Could you check a few things on this model? Use its own coordinates, in mm. A direction names the side the tool comes from. Coordinates: 2 decimals unless noted, no trailing zeros. Order: outer loops, then holes, each group sorted by start corner. A loop starts at its lowest first (then second) coordinate and runs counter-clockwise, first axis right, second up. Notation, with made-up numbers: (-30, 66) - (5, 66) arc R24 ccw to (5, 101) - close; hole circle Ø7 at (79.25, 70). An arc over 180 degrees is marked (long way). One line per item, written item: value. Start each with the question number.
from build123d import *

# Parameters (mm, degrees)
SKETCH1_W             = 15
SKETCH1_H             = 15
BOSS_EXTRUDE1_DEPTH   = 10
SKETCH2_R             = 6
CUT_EXTRUDE1_DEPTH    = 4
SKETCH3_R             = 5
CUT_EXTRUDE2_DEPTH    = 3.5
BOSS_EXTRUDE2_DEPTH   = 6.5
M4_TAPPED_HOLE1_D     = 3.3
M4_TAPPED_HOLE1_DEPTH = 2.5
M2_5_TAPPED_HOLE1_D   = 2.05
SKETCH10_R            = 0.25
CUT_EXTRUDE3_DEPTH    = 0.25
CUT_EXTRUDE4_REACH    = 23.5


with BuildPart() as part:
    # Sketch1 → Boss-Extrude1 (new body)
    with BuildSketch(Plane(origin=(0, 0, 0), x_dir=(1, 0, 0), z_dir=(0, 1, 0))):
        Rectangle(SKETCH1_W, SKETCH1_H)
    extrude(amount=BOSS_EXTRUDE1_DEPTH)

    # Sketch2 → Cut-Extrude1 (cut)
    with BuildSketch(Plane.XZ):
        Circle(SKETCH2_R)
    extrude(amount=-CUT_EXTRUDE1_DEPTH, mode=Mode.SUBTRACT)

    # Sketch3 → Cut-Extrude2 (cut)
    with BuildSketch(Plane.XZ.offset(-4)):
        Circle(SKETCH3_R)
    extrude(amount=-CUT_EXTRUDE2_DEPTH, mode=Mode.SUBTRACT)

    # Sketch4 → Boss-Extrude2 (add)
    with BuildSketch(Plane.XY.offset(7.5)):
        with BuildLine():
            ThreePointArc((5.823428515, 4.483331092), (0, 5.25), (-5.823428515, 4.483331092))
            ThreePointArc((-5.823428515, 4.483331092), (-6.707311991, 2.952400002), (-5.176380902, 2.068516526))
            ThreePointArc((-5.176380902, 2.068516526), (0, 2.75), (5.176380902, 2.068516526))
            ThreePointArc((5.176380902, 2.068516526), (6.707311991, 2.952400002), (5.823428515, 4.483331092))
        make_face()
    boss_extrude2 = extrude(amount=BOSS_EXTRUDE2_DEPTH)

    # Mirror1: Boss-Extrude2 across plane
    add(boss_extrude2.mirror(Plane.XY))

    # M4 Tapped Hole1
    with Locations(Plane(origin=(0, 10, 0), x_dir=(1, 0, 0), z_dir=(0, 1, 0))):
        with Locations((0, 0)):
            Hole(M4_TAPPED_HOLE1_D / 2, depth=M4_TAPPED_HOLE1_DEPTH)

    # M2.5 Tapped Hole1 (through all)
    with Locations(Plane(origin=(0, 10, 0), x_dir=(1, 0, 0), z_dir=(0, 1, 0))):
        with Locations((0, 11.5), (0, -11.5)):
            Hole(M2_5_TAPPED_HOLE1_D / 2)

    # Sketch10 → Cut-Extrude3 (cut)
    with BuildSketch(Plane.XY.offset(14)):
        with Locations((-5.499904708, 3.275923809)):
            Circle(SKETCH10_R)
        with Locations((5.499904708, 3.275923809)):
            Circle(SKETCH10_R)
    extrude(amount=-CUT_EXTRUDE3_DEPTH, mode=Mode.SUBTRACT)

    # Sketch11 → Cut-Extrude4 (cut, up to next)
    with BuildSketch(Plane.XY.offset(7.5), mode=Mode.PRIVATE) as cut_extrude4_sk1:
        Polygon((-7.5, 10), (-6.395762797, 0), (-7.5, 0), align=None)
    cut_extrude4_tool1 = extrude(cut_extrude4_sk1.sketch, amount=-CUT_EXTRUDE4_REACH, mode=Mode.PRIVATE) & part.part
    add(cut_extrude4_tool1.solids().sort_by_distance((-7.131921, 3.333333, 7.5))[0], mode=Mode.SUBTRACT)
    # Sketch11 → Cut-Extrude4 (cut, up to next)
    with BuildSketch(Plane.XY.offset(7.5), mode=Mode.PRIVATE) as cut_extrude4_sk2:
        Polygon((7.5, 10), (6.395762797, 0), (7.5, 0), align=None)
    cut_extrude4_tool2 = extrude(cut_extrude4_sk2.sketch, amount=-CUT_EXTRUDE4_REACH, mode=Mode.PRIVATE) & part.part
    add(cut_extrude4_tool2.solids().sort_by_distance((7.131921, 3.333333, 7.5))[0], mode=Mode.SUBTRACT)


solid = part.part
Q1. We'd pull the mould along X, two halves only. Please class faces 1 (the cylindrical face through (-6, 2, 0)), 2 (the flat face through (-6.956, 5.07, 0.105)), 3 (the flat face through (-6, 0, -2)), 4 (the cylindrical face through (-0.07, 2.75, 9.98)): +X half, -X half, draft (parallel to the pull), parting line (faces both ways), or undercut.
Q2. I'm going to push flat-ended pins straight in: pin 1 (8 mm diameter, centred on x = 0, z = 0, fed in from -Y); pin 2 (2.5 mm diameter, centred on x = 0, z = 11.5, fed in from -Y); pin 3 (1 mm diameter, centred on y = 4, z = -1.5, fed in from +X); pin 4 (1 mm diameter, centred on x = -1, z = 0, fed in from +Y). Where does each tip first touch, or does it pass through?
Q3. If I drill on L1, parallel to Z at x = 0, y = 4.4 (3 decimals); L2, parallel to Z at x = 0, y = 2.4; L3, parallel to Z at x = -7, y = 9.25, over which ranges is the centre line in solid material (lowest first)?
Q4. Which directions (+Z, -Z, +X, -X, +Y, -Y) give clear straight access to the entire face, cutting with the end or side of a thin tool? Please do faces 5 (the flat face through (-4, 4, 4)), 6 (the cylindrical face through (-0.07, 2.75, -9.98)), 7 (the flat face through (0, 1, 7.5)), 8 (the cylindrical face through (0.76, 3.97, 10.81)).
Q5. I want a section at A-A on x = 0. State how many separate pieces and enclosed holes the cut face has, then the cut area to 3 significant figures.
Q6. I want a section at C-C on y = 8. Please give me the cut outline in (x, z), then the cut area to 3 significant figures.
Q7. I want a section at D-D on z = -2.5. Please give me the cut outline in (x, y), then the cut area to 3 significant figures.
Values follow:
1. face 1: undercut
1. face 2: -X half
1. face 3: draft
1. face 4: undercut
2. pin 1: stops at y = 7.5
2. pin 2: stops at y = 2.71
2. pin 3: stops at x = 6.89
2. pin 4: passes through
3. L1: z = -14 to -12.525, -10.475 to -5, 5 to 10.475, 12.525 to 14
3. L2: z = -7.5 to -6, 6 to 7.5
3. L3: z = -7.5 to 7.5
4. face 5: -Y
4. face 6: -Z, -Y
4. face 7: +Z, -Y
4. face 8: +Y, -Y
5. separate pieces: 4
5. enclosed holes: 0
5. area: 81.0 mm^2
6. outline: (-7.28, -7.5) - (7.28, -7.5) - (7.28, 7.5) - (-7.28, 7.5) - close; hole circle Ø3.3 at (0, 0)
6. area: 210 mm^2
7. outline: (-7.5, 10) - (-6.4, 0) - (-5.45, 0) - (-5.45, 4) - (-4.33, 4) - (-4.33, 7.5) - (4.33, 7.5) - (4.33, 4) - (5.45, 4) - (5.45, 0) - (6.4, 0) - (7.5, 10) - close
7. area: 65.0 mm^2
